from build123d import *

# Parameters (mm, degrees)
CROQUIS1_R              = 14.493410581
SALIENTE_EXTRUIR1_DEPTH = 30
CROQUIS2_R              = 6.849720654
SALIENTE_EXTRUIR2_DEPTH = 60


with BuildPart() as part:
    # Croquis1 → Saliente-Extruir1 (new body)
    with BuildSketch(Plane(origin=(0, 0, 0), x_dir=(0, 0, -1), z_dir=(1, 0, 0))):
        Polygon((25, 14.43375673), (0, 28.867513459), (-25, 14.43375673), (-25, -14.43375673), (0, -28.867513459), (25, -14.43375673), align=None)
        Circle(CROQUIS1_R, mode=Mode.SUBTRACT)
    extrude(amount=SALIENTE_EXTRUIR1_DEPTH)

    # Croquis2 → Saliente-Extruir2 (add)
    with BuildSketch(Plane(origin=(0, 0, -25), x_dir=(-1, 0, 0), z_dir=(0, 0, -1))):
        with Locations(Location((-14.099346636, 0, 0), (0, 0, 180))):
            Circle(CROQUIS2_R)
    extrude(amount=SALIENTE_EXTRUIR2_DEPTH)


solid = part.part
Verification items for the finished model (mm, model axes). Coordinates: 2 decimals unless noted, no trailing zeros. Loops run counter-clockwise (first coordinate to the right, second up) from the corner with the lowest first, then second, coordinate; pieces in that order, holes last. Notation, with made-up numbers: (30.5, 86) -> (53.5, 86) arc R15 ccw to (53.5, 91) -> close; hole circle Ø6 at (-15, -30.75). An arc over 180 degrees is marked (long way). Answer as CSV lines item,"result".
1) Cross-section at D-D, the plane z = -34. Record the cut outline in (x, y), then the cut area to 3 significant figures.
Found:
outline,"circle Ø13.7 at (14.1, 0)"
area,"147 mm2"
2) Cross-section at B-B, the plane z = -8. Record the cut outline in (x, y).
Found:
outline,"(0, -24.25) -> (30, -24.25) -> (30, -12.09) -> (0, -12.09) -> close; (0, 12.09) -> (30, 12.09) -> (30, 24.25) -> (0, 24.25) -> close"
3) Thickness scan on L1, parallel to Y at x = 24, z = 0; L2, parallel to Z at x = 27.25, y = 1.5; L3, parallel to Z at x = 11.75, y = 4. Record the ranges inside material, lowest first. Write a range as from..to.
Found:
L1,"y = -28.87..-14.49, 14.49..28.87"
L2,"z = -25..-14.42, 14.42..25"
L3,"z = -85..-13.93, 13.93..25"
4) Cross-section at C-C, the plane y = 0. Record the cut outline in (x, z), then the cut area to 3 significant figures.
Found:
outline,"(0, -25) -> (7.25, -25) -> (7.25, -85) -> (20.95, -85) -> (20.95, -25) -> (30, -25) -> (30, -14.49) -> (0, -14.49) -> close; (0, 14.49) -> (30, 14.49) -> (30, 25) -> (0, 25) -> close"
area,"1,450 mm2"
5) Release check for a two-part mould opening along Z. For faces 1 (the flat face through (21.5, -0.2, -25)), 2 (the cylindrical face through (7.256, -0.301, -54.58)), 3 (the cylindrical face through (14.79, -14.15, 3.14)) record: +Z half, -Z half, draft (parallel to the pull), parting line (faces both ways), or undercut.
Found:
face 1,"-Z half"
face 2,"draft"
face 3,"undercut"
6) Depth check by flat-ended pin: pin 1 (1 mm diameter, centred on y = -19.5, z = -1.5, fed in from -X); pin 2 (12 mm diameter, centred on x = 7.5, z = -8, fed in from -Y); pin 3 (12 mm diameter, centred on x = 24.5, z = -24, fed in from -Y); pin 4 (8 mm diameter, centred on x = 23, y = 16.5, fed in from -Z). Enter the tip coordinate at first touch or a pass-through.
Found:
pin 1,"stops at x = 0"
pin 2,"stops at y = -27.71"
pin 3,"stops at y = -18.48"
pin 4,"stops at z = -25"
7) Cross-section at A-A, the plane x = 3.75. Record the cut outline in (y, z), then the cut area to 3 significant figures.
Found:
outline,"(-28.87, 0) -> (-14.43, -25) -> (14.43, -25) -> (28.87, 0) -> (14.43, 25) -> (-14.43, 25) -> close; hole circle Ø28.99 at (0, 0)"
area,"1,510 mm2"
